from build123d import *

# Parameters (mm, degrees)
ESBO_O1_W                     = 50
ESBO_O1_H                     = 80
RESSALTO_EXTRUS_O1_DEPTH      = 5
ESBO_O2_W                     = 42.3
ESBO_O2_H                     = 42.3
CORTE_EXTRUS_O1_DEPTH         = 2
ESBO_O3_R                     = 11.02
CORTE_EXTRUS_O2_DEPTH         = 24
ESBO_O4_R                     = 1.987893006
CORTE_EXTRUS_O3_DEPTH         = 24
PADR_OCIRCULAR1_COUNT         = 4
ESBO_O5_R                     = 4
CORTE_EXTRUS_O4_DEPTH         = 24
CHANFRO1_SIZE                 = 5.6
ESBO_O6_R                     = 1.75
CORTE_EXTRUS_O5_DEPTH         = 10
FILETE1_R                     = 2
ESBO_O7_W                     = 30
ESBO_O7_H                     = 10
RESSALTO_EXTRUS_O2_DEPTH      = 50
RESSALTO_EXTRUS_O2_DEPTH_BACK = 10
ESBO_O8_R                     = 4.05
CORTE_EXTRUS_O6_DEPTH         = 45
ESBO_O9_W                     = 12
ESBO_O9_H                     = 50
CORTE_EXTRUS_O7_DEPTH         = 45
FILETE2_R                     = 10
FILETE3_R                     = 8


with BuildPart() as part:
    # Esboço1 → Ressalto-extrusão1 (new body, symmetric)
    with BuildSketch(Plane.XY):
        Rectangle(ESBO_O1_W, ESBO_O1_H)
    extrude(amount=RESSALTO_EXTRUS_O1_DEPTH, both=True)

    # Esboço2 → Corte-extrusão1 (cut)
    with BuildSketch(Plane.XY.offset(5)):
        Rectangle(ESBO_O2_W, ESBO_O2_H)
    extrude(amount=-CORTE_EXTRUS_O1_DEPTH, mode=Mode.SUBTRACT)

    # Esboço3 → Corte-extrusão2 (cut)
    with BuildSketch(Plane.XY.offset(3)):
        Circle(ESBO_O3_R)
    extrude(amount=-CORTE_EXTRUS_O2_DEPTH, mode=Mode.SUBTRACT)

    # Esboço4 → Corte-extrusão3 (cut)
    with BuildSketch(Plane.XY.offset(3)):
        with Locations((-15.59, 15.5)):
            Circle(ESBO_O4_R)
    corte_extrus_o3 = extrude(amount=-CORTE_EXTRUS_O3_DEPTH, mode=Mode.SUBTRACT)

    # PadrãoCircular1: Corte-extrusão3 ×4 about axis
    padr_ocircular1_axis = Axis((0, 0, 0), (0, 0, 1))
    for i in range(1, PADR_OCIRCULAR1_COUNT):
        add(corte_extrus_o3.rotate(padr_ocircular1_axis, i * 360 / PADR_OCIRCULAR1_COUNT), mode=Mode.SUBTRACT)

    # Esboço5 → Corte-extrusão4 (cut)
    with BuildSketch(Plane.XY.offset(5)):
        with Locations((0, 27)):
            Circle(ESBO_O5_R)
        with Locations((0, -27)):
            Circle(ESBO_O5_R)
    extrude(amount=-CORTE_EXTRUS_O4_DEPTH, mode=Mode.SUBTRACT)

    # Chanfro1
    chanfro1_edges = [part.edges().sort_by_distance(p)[0] for p in [
        (21.15, 21.15, 4),
        (21.15, -21.15, 4),
        (-21.15, -21.15, 4),
        (-21.15, 21.15, 4),
    ]]
    chamfer(chanfro1_edges, length=CHANFRO1_SIZE)

    # Esboço6 → Corte-extrusão5 (cut)
    with BuildSketch(Plane(origin=(0, 0, -5), x_dir=(-1, 0, 0), z_dir=(0, 0, -1))):
        with Locations((-17, 32)):
            Circle(ESBO_O6_R)
        with Locations((17, 32)):
            Circle(ESBO_O6_R)
        with Locations((-17, -32)):
            Circle(ESBO_O6_R)
        with Locations((17, -32)):
            Circle(ESBO_O6_R)
    extrude(amount=-CORTE_EXTRUS_O5_DEPTH, mode=Mode.SUBTRACT)

    # Filete1
    filete1_edges = [part.edges().sort_by_distance(p)[0] for p in [
        (25, -40, 0),
        (-25, 40, 0),
        (25, 40, 0),
    ]]
    fillet(filete1_edges, radius=FILETE1_R)

    # Esboço7 → Ressalto-extrusão2 (add, two sides)
    with BuildSketch(Plane(origin=(0, 0, -5), x_dir=(-1, 0, 0), z_dir=(0, 0, -1))) as ressalto_extrus_o2_sk:
        with Locations((40, -35)):
            Rectangle(ESBO_O7_W, ESBO_O7_H)
    extrude(amount=RESSALTO_EXTRUS_O2_DEPTH)
    extrude(ressalto_extrus_o2_sk.sketch, amount=-RESSALTO_EXTRUS_O2_DEPTH_BACK)

    # Esboço8 → Corte-extrusão6 (cut)
    with BuildSketch(Plane(origin=(0, -40, 0), x_dir=(-1, 0, 0), z_dir=(0, -1, 0))):
        with Locations((46, 45.5)):
            Circle(ESBO_O8_R)
    extrude(amount=-CORTE_EXTRUS_O6_DEPTH, mode=Mode.SUBTRACT)

    # Esboço9 → Corte-extrusão7 (cut)
    with BuildSketch(Plane(origin=(0, -40, 0), x_dir=(-1, 0, 0), z_dir=(0, -1, 0))):
        with Locations((31, 30)):
            Rectangle(ESBO_O9_W, ESBO_O9_H)
    extrude(amount=-CORTE_EXTRUS_O7_DEPTH, mode=Mode.SUBTRACT)

    # Filete2
    filete2_edges = [part.edges().sort_by_distance(p)[0] for p in [
        (-55, -35, 5),
        (-37, -35, -5),
    ]]
    fillet(filete2_edges, radius=FILETE2_R)

    # Filete3
    filete3_edges = [part.edges().sort_by_distance(p)[0] for p in [
        (-25, -30, 0),
    ]]
    fillet(filete3_edges, radius=FILETE3_R)


solid = part.part
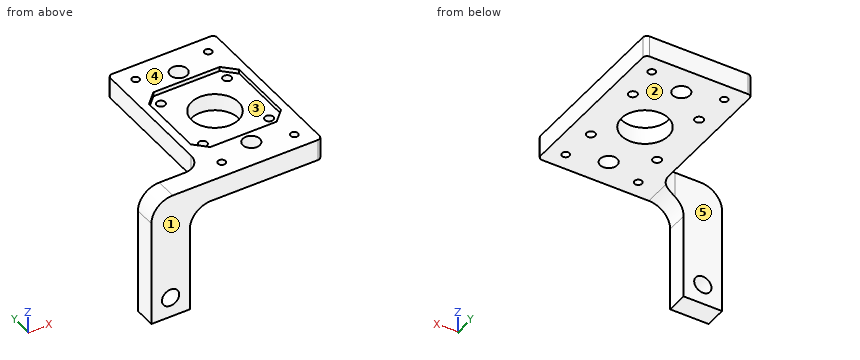
Model file for the job. Use its own axes, mm. Face numbers are marked on the shaded views. A direction names the side the tool comes from. Round coordinates to 2 decimals unless told otherwise and drop trailing zeros. Order: outer loops, then holes, each group sorted by start corner. A loop starts at its lowest first (then second) coordinate and runs counter-clockwise, first axis right, second up. Notation, with made-up numbers: M -16.5,72 L 24.5,72 A20 ccw 24.5,102 Z; hole C -31,66 d7. An arc over 180 degrees is marked long. Write each question's results on one line, items separated by ' | '. Start each with the question number.
(1) Which spindle directions (+Z, -Z, +X, -X, +Y, -Y) get a long thin tool onto all of the face, cutting with end or side? Do the marked faces 1 and 2. Say none if no direction does.
(2) Drop flat-ended pins along their axis: pin 1 (7 mm diameter, centred on x = 0, y = 27, fed in from +Z); pin 2 (5.5 mm diameter, centred on x = 17, y = -32, fed in from -Z); pin 3 (4.5 mm diameter, centred on x = 15.5, y = 15.59, fed in from +Z); pin 4 (24 mm diameter, centred on x = -42.5, z = -31, fed in from +Y). Give the stop position or say it passes through.
(3) Saw through at A-A, the plane z = -45.5. Give the cut face in (x, y), then the cut area to 3 significant figures.
(4) Saw through at B-B, the plane y = 27. Give the cut face in (x, z).
(5) Saw through at D-D, the plane z = -23.5. Give the cut face in (x, y).
(6) Saw through at C-C, the plane x = 20. Give the cut face in (y, z).
(7) Probe probe 1 along X at (y, z) = (15.59, -0.25); probe 2 along Y at (x, z) = (-15.5, -0.5); probe 3 along Y at (x, z) = (17, 1). List the from-to ranges inside material, lowest first. Write a range as from..to.
(8) Two-plate mould, pull along Y, no slides. Class the marked faces 3, 4 and 5: pulls with the +Y half, pulls with the -Y half, needs draft (parallel to the pull), parting line crosses it, or undercut.
Established:
1) face 1: +Z, -Z, +X, -X, -Y | face 2: -Z, +X, +Y, -Y
2) pin 1: passes through | pin 2: stops at z = -5 | pin 3: stops at z = 3 | pin 4: stops at y = -30
3) outline: M -55,-40 L -50.05,-40 L -50.05,-30 L -55,-30 Z; M -41.95,-40 L -37,-40 L -37,-30 L -41.95,-30 Z | area: 99.0 mm^2
4) outline: M -25,-5 L -4,-5 L -4,5 L -25,5 Z; M 4,-5 L 25,-5 L 25,5 L 4,5 Z
5) outline: M -55,-40 L -37,-40 L -37,-30 L -55,-30 Z
6) outline: M -40,-5 L 40,-5 L 40,5 L 16.7,5 L 16.7,3 L -16.7,3 L -16.7,5 L -40,5 Z
7) probe 1: x = -25..-17.58, -13.6..13.51, 17.49..25 | probe 2: y = -40..-32.9, -31.1..-17.58, -13.6..13.51, 17.49..31.1, 32.9..40 | probe 3: y = -40..-33.75, -30.25..-16.9, -14.1..14.29, 16.89..30.25, 33.75..40
8) face 3: undercut | face 4: needs draft | face 5: pulls with the +Y half
